Autodesk Inventor part; units mm, degrees
ref_plane "YZ Plane" through (0, 0, 0) normal (1, 0, 0) x (0, 1, 0)
ref_plane "XZ Plane" through (0, 0, 0) normal (0, 1, 0) x (-1, 0, 0)
ref_plane "XY Plane" through (0, 0, 0) normal (0, 0, 1) x (1, 0, 0)
sketch "Sketch1" plane through (0, 0, 0) normal (0, 1, 0) x (-1, 0, 0)
  line L0 (0, 0) -> (38.1, 0)
  line L1 (38.1, 0) -> (38.1, -19.05)
  line L2 (38.1, -19.05) -> (0, -19.05)
  line L3 (0, -19.05) -> (0, 0)
  line L4 (38.1, -19.05) -> (32.512, -19.05)
  line L5 (32.512, -19.05) -> (32.512, 0)
  line L6 (32.512, 0) -> (38.1, 0)
  line L7 (38.1, 0) -> (38.1, -19.05)
  line L8 (0, -19.05) -> (5.588, -19.05)
  line L9 (5.588, -19.05) -> (5.588, 0)
  line L10 (5.588, 0) -> (0, 0)
  line L11 (0, 0) -> (0, -19.05)
  point P0 (5.588, -19.05)
  dimension "d0" = 38.1
  dimension "d1" = 19.05
  dimension "d2" = 5.588
  dimension "d3" = 5.588
extrude "Extrusion1" add sketch "Sketch1" along normal blind 25.4 contours L0 L9 L2 L3 | L0 L1 L2 L5
extrude "Extrusion2" add sketch "Sketch1" against normal blind 5.08
sketch "Sketch2" plane through (0, 25.4, 0) normal (1, 0, 0) x (0, 0, -1)
  line L0 (19.05, 0) -> (0, 0)
  line L1 (9.525, 0) -> (9.525, -12.7)
  point P0 (0, -25.4)
  dimension "d8" = 12.7
hole "Hole1" at (0, 12.7, -9.525) direction (-1, 0, 0) diameter 6.7564 end through all
sketch "Sketch3" plane through (0, -5.08, 0) normal (0, -1, 0) x (1, 0, 0)
  line L0 (0, 0) -> (-38.1, 0)
  line L1 (-38.1, 0) -> (-35.56, 0)
  line L2 (-35.56, 0) -> (-35.56, -2.54)
  line L3 (-35.56, -2.54) -> (-38.1, -2.54)
  line L4 (-38.1, -2.54) -> (-38.1, 0)
  line L5 (0, -19.05) -> (-2.54, -19.05)
  line L6 (-2.54, -19.05) -> (-2.54, -16.51)
  line L7 (-2.54, -16.51) -> (0, -16.51)
  line L8 (0, -16.51) -> (0, -19.05)
  line L9 (-35.56, -2.54) -> (-2.54, -2.54)
  line L10 (-2.54, -2.54) -> (-2.54, -16.51)
  line L11 (-2.54, -16.51) -> (-35.56, -16.51)
  line L12 (-35.56, -16.51) -> (-35.56, -2.54)
  line L13 (-38.1, 0) -> (-38.1, -19.05)
  line L14 (0, -19.05) -> (0, 0)
  line L15 (-38.1, -19.05) -> (0, -19.05)
  dimension "d16" = 2.54
  dimension "d17" = 2.54
  dimension "d18" = 2.54
  dimension "d19" = 2.54
extrude "Extrusion3" cut sketch "Sketch3" against normal blind 2.54 contours L9 L10 L11 L12
extrude "Extrusion4" add sketch "Sketch3" along normal blind 8.255 contours L14 L7 L10 L9 L2 L0 | L2 L3 L4 L0 | L8 L5 L6 L7 | L12 L11 L6 L15 L13 L3
sketch "Sketch4" plane through (0, 25.4, 0) normal (1, 0, 0) x (0, 0, -1)
  line L0 (19.05, -38.735) -> (19.05, 0)
  line L1 (19.05, -30.3802) -> (6.35, -30.3802)
  line L2 (19.05, -30.3802) -> (31.75, -30.3802) construction
  point P0 (0, -25.4)
  dimension "d24" = 12.7
  dimension "d25" = 180
hole "Hole2" at (0, -4.9802, -6.35) direction (-1, 0, 0) diameter 3.4544 depth 2.54
sketch "Sketch5" plane through (0, -2.54, 0) normal (0, -1, 0) x (1, 0, 0)
  line L0 (-2.54, -16.51) -> (-35.56, -16.51)
  line L1 (-19.05, -16.51) -> (-19.05, -2.54)
  line L2 (-35.56, -2.54) -> (-2.54, -2.54)
  line L3 (-35.56, -2.54) -> (-2.54, -2.54)
  line L4 (-19.05, -16.51) -> (-19.05, -9.525)
  line L5 (-4.2545, -5.715) -> (-33.8455, -5.715)
  line L6 (-33.8455, -5.715) -> (-33.8455, -13.335)
  line L7 (-33.8455, -13.335) -> (-4.2545, -13.335)
  line L8 (-4.2545, -13.335) -> (-4.2545, -5.715)
  line L9 (-4.2545, -5.715) -> (-33.8455, -13.335) construction
  line L10 (-33.8455, -5.715) -> (-4.2545, -13.335) construction
  line L11 (-19.05, -9.525) -> (-30.4165, -9.525)
  line L12 (-30.4165, -9.525) -> (-7.6835, -9.525)
  point P0 (0, 0)
  dimension "d33" = 6.985
  dimension "d34" = 29.591
  dimension "d35" = 7.62
  dimension "d36" = 11.3665
  dimension "d37" = 22.733
hole "Hole3" at (-7.6835, -2.54, -9.525) at (-30.4165, -2.54, -9.525) direction (0, 1, 0) diameter 2.2606 end through all
sketch "Sketch6" plane through (-35.56, -2.54, -16.51) normal (0, 0, 1) x (1, 0, 0)
  line L0 (33.02, 0) -> (0, 0)
  line L1 (16.51, 0) -> (16.51, -10.541)
  point P0 (35.56, 2.54)
  dimension "d45" = 10.541
hole "Hole4" at (-19.05, -13.081, -16.51) direction (0, 0, 1) diameter 3.302 end through all both
fillet "Fillet1" radius 3.175 6 edges at (-38.1, 6.0325, 0) (0, 6.0325, 0) (0, 6.0325, -19.05) (0, 25.4, -9.525) (-38.1, 6.0325, -19.05) (-38.1, 25.4, -9.525)
properties part number "HomemadeSensorHousing 8020"
Geometry: final body of the model. Coordinates: model frame, mm. A direction names the side the tool comes from. Round coordinates to 2 decimals unless told otherwise and drop trailing zeros. Order: outer loops, then holes, each group sorted by start corner. A loop starts at its lowest first (then second) coordinate and runs counter-clockwise, first axis right, second up. Notation, with made-up numbers: (42, -14.5) -> (55, -14.5) arc R27 ccw to (55, 3.5) -> close; hole circle Ø2 at (33, -12.5). An arc over 180 degrees is marked (long way). Use one line per item in the form item = value. Start each with the question number.
1. Cut plane B-B (x = -33). Return the cut outline in (y, z) (3 decimals).
2. Cut plane A-A (y = 12.7). Return the cut outline in (x, z) (3 decimals).
3. Reachability of faces 1 (the face through (-19, -3, 0)), 2 (the face through (-1.288, -6.693, -6.125)), 3 (the face through (-19, 0, -9)), 4 (the face through (-19, -8, -16.51)), 5 (the face through (-37.15, 5.76, -0.91)) from +Z, -Z, +X, -X, +Y, -Y: full face, straight path, thin tool, end or side. Return the list, or none.
4. Pin query (flat end, axial travel): pin 1 Ø5.5 at (y, z) = (12.7, -9.525) entering from -X; pin 2 Ø3.5 at (x, z) = (-7.68, -9.52) entering from +Y; pin 3 Ø8 at (x, z) = (-21.5, -7.5) entering from -Y. Return the tip coordinate at first contact, or that it passes through.
5. Cut plane D-D (y = 8.5). Return the cut outline in (x, z) (3 decimals).
6. Draft query along X for faces 6 (the face through (-5.588, 10, -12)), 7 (the face through (-37.19, 5.76, -18.1)), 8 (the face through (-4, 25.4, -9)). Return one class per face: pulls with the +X half, pulls with the -X half, needs draft (parallel to the pull), parting line crosses it, or undercut.
7. Cut plane C-C (y = -10). Return the cut outline in (x, z) (3 decimals), then the cut area to 3 significant figures.
8. Line query: probe 1 along X at (y, z) = (-3.5, -10.75); probe 2 along Z at (x, y) = (-9.5, -10); probe 3 along X at (y, z) = (19, -15.75). Output: solid intervals per line, ascending.
Solution:
q1.outline = (-13.335, -19.05) -> (25.4, -19.05) -> (25.4, 0) -> (-13.335, 0) -> (-13.335, -2.54) -> (-2.54, -2.54) -> (-2.54, -16.51) -> (-13.335, -16.51) -> close; hole circle Ø6.756 at (12.7, -9.525)
q2.outline = (-38.1, -15.875) arc R3.175 ccw to (-34.925, -19.05) -> (-32.512, -19.05) -> (-32.512, -12.903) -> (-38.1, -12.903) -> close; (-38.1, -6.147) -> (-32.512, -6.147) -> (-32.512, 0) -> (-34.925, 0) arc R3.175 ccw to (-38.1, -3.175) -> close; (-5.588, -19.05) -> (-3.175, -19.05) arc R3.175 ccw to (0, -15.875) -> (0, -12.903) -> (-5.588, -12.903) -> close; (-5.588, -6.147) -> (0, -6.147) -> (0, -3.175) arc R3.175 ccw to (-3.175, 0) -> (-5.588, 0) -> close
q3.face_1 = +Z, +X, -X, +Y, -Y
q3.face_2 = +X
q3.face_3 = +Z, -Z, +Y
q3.face_4 = -Y
q3.face_5 = +Z, -X, +Y, -Y
q4.pin_1 = through
q4.pin_2 = 0
q4.pin_3 = -2.54
q5.outline = (-38.1, -15.875) arc R3.175 ccw to (-34.925, -19.05) -> (-32.512, -19.05) -> (-32.512, 0) -> (-34.925, 0) arc R3.175 ccw to (-38.1, -3.175) -> close; (-5.588, -19.05) -> (-3.175, -19.05) arc R3.175 ccw to (0, -15.875) -> (0, -3.175) arc R3.175 ccw to (-3.175, 0) -> (-5.588, 0) -> close
q6.face_6 = undercut
q6.face_7 = pulls with the -X half
q6.face_8 = needs draft
q7.outline = (-38.1, -15.875) arc R3.175 ccw to (-34.925, -19.05) -> (-3.175, -19.05) arc R3.175 ccw to (0, -15.875) -> (0, -3.175) arc R3.175 ccw to (-3.175, 0) -> (-34.925, 0) arc R3.175 ccw to (-38.1, -3.175) -> close; hole (-35.56, -16.51) -> (-2.54, -16.51) -> (-2.54, -2.54) -> (-35.56, -2.54) -> close
q7.area = 256 mm^2
q8.probe_1 = -38.1 to -35.56, -2.54 to 0
q8.probe_2 = -19.05 to -16.51, -2.54 to 0
q8.probe_3 = -38.1 to -32.51, -5.59 to 0
